from build123d import *

# Parameters (mm, degrees)
F0_R     = 27
F0_R_2   = 25
F1_DEPTH = 1
F2_DEPTH = 8
F3_R     = 20
F4_DEPTH = 7


with BuildPart() as f1:
    # F0 (on Top) → F1 (new body)
    with BuildSketch(Plane.XY):
        Circle(F0_R)
        Circle(F0_R_2, mode=Mode.SUBTRACT)
        Circle(F0_R_2)
    extrude(amount=F1_DEPTH)

    # F0 (on Top) → F2 (join)
    with BuildSketch(Plane.XY):
        Circle(F0_R_2)
    extrude(amount=F2_DEPTH)

    # F3 (on face) → F4 (cut)
    with BuildSketch(Plane.XY.offset(8)):
        Circle(F3_R)
    extrude(amount=-F4_DEPTH, mode=Mode.SUBTRACT)


solid = f1.part
Build history of the part. All positions in model axes, mm. A direction names the side the tool comes from. Coordinates: 2 decimals unless noted, no trailing zeros. Order: outer loops, then holes, each group sorted by start corner. A loop starts at its lowest first (then second) coordinate and runs counter-clockwise, first axis right, second up. Notation, with made-up numbers: (61.25, 61) - (85.25, 61) arc R27 ccw to (85.25, 83) - close; hole circle Ø5 at (11, 49). An arc over 180 degrees is marked (long way). Write item = value, one per line. Start each with the question number.
1) Flat gauge pins, fed straight in: pin 1 Ø1 at (y, z) = (21.5, 5) entering from -X; pin 2 Ø1.5 at (y, z) = (-19.5, 3.5) entering from +X; pin 3 Ø1.5 at (x, z) = (4.5, 4) entering from +Y. Where does each tip first touch, or does it go through?
2) Wall check: line 1 along Y through (x, z) = (0, 4.75); line 2 along Z through (x, y) = (4, -3); line 3 along Y through (x, z) = (-5.5, 7.25). Give the ranges that are in metal, low to high. Write a range as from..to.
3) Saw through at C-C on y = -9. Write the cut outline in (x, z).
4) Two-plate mould, pull along Y, no slides. Class faces 1 (the face through (0, 0, 0)), 2 (the face through (0, 0, 1)), 3 (the face through (23.846, 7.509, 4.451)): pulls with the +Y half, pulls with the -Y half, needs draft (parallel to the pull), parting line crosses it, or undercut.
5) Saw through at A-A on z = 2.75. Write the cut outline in (x, y).
6) Saw through at B-B on x = 0. Write the cut outline in (y, z), then the cut area to 3 significant figures.
7) 3-axis set-ups, long thin cutter, end or side, ignore diameter. For faces 4 (the face through (24, -8, 1)), 5 (the face through (-5.85, -26.36, 0.49)): which of +Z, -Z, +X, -X, +Y, -Y reach the whole face in a straight line?
From the geometry:
q1.pin_1 = -13.56
q1.pin_2 = 16.54
q1.pin_3 = 24.72
q2.line_1 = -25..-20, 20..25
q2.line_2 = 0..1
q2.line_3 = -24.39..-19.23, 19.23..24.39
q3.outline = (-25.46, 0) - (25.46, 0) - (25.46, 1) - (23.32, 1) - (23.32, 8) - (17.86, 8) - (17.86, 1) - (-17.86, 1) - (-17.86, 8) - (-23.32, 8) - (-23.32, 1) - (-25.46, 1) - close
q4.face_1 = needs draft
q4.face_2 = undercut
q4.face_3 = parting line crosses it
q5.outline = circle Ø50 at (0, 0); hole circle Ø40 at (0, 0)
q6.outline = (-27, 0) - (27, 0) - (27, 1) - (25, 1) - (25, 8) - (20, 8) - (20, 1) - (-20, 1) - (-20, 8) - (-25, 8) - (-25, 1) - (-27, 1) - close
q6.area = 124 mm^2
q7.face_4 = +Z
q7.face_5 = +Z, -Z
